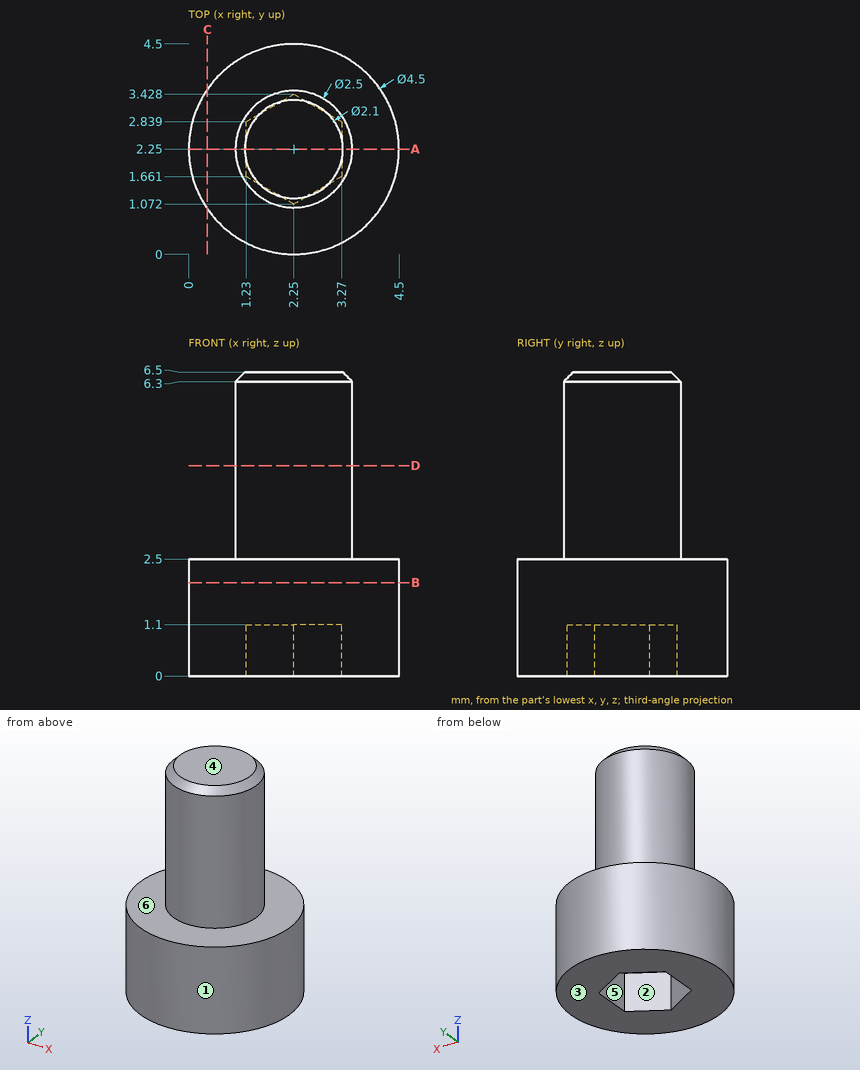
Can you work these out from the drawing? Everything is in mm from the part's minimum corner. A direction names the side the tool comes from. Round coordinates to 2 decimals unless told otherwise and drop trailing zeros. Write each loop counter-clockwise with the first axis right and the second up, starting at its lowest first coordinate (ties: lowest second). Pieces come first, ordered by that corner, then holes. Notation, with made-up numbers: (2, 63.5) - (28, 63.5) arc R24 ccw to (28, 75.5) - close; hole circle Ø10 at (-39.75, 57). An arc over 180 degrees is marked (long way). Write each question's results on one line, items separated by ' | '. Start each with the question number.
1) Suppose I cut it at B-B (z = 2). List the corners of the cut face in (x, y) for me.
2) Suppose I cut it at A-A (y = 2.25). List the corners of the cut face in (x, z) for me.
3) Suppose I cut it at D-D (z = 4.5). List the corners of the cut face in (x, y) for me, and give its area (3 significant figures).
4) Which directions (+Z, -Z, +X, -X, +Y, -Y) give clear straight access to the entire face, cutting with the end or side of a thin tool? Please do the marked faces 4, 5 and 6.
5) Please list where these lines run through material, in increasing order: line 1 (Y direction, x = 1.6, z = 1); line 2 (Z direction, x = 3.8, y = 3); line 3 (X direction, y = 1.95, z = 0.5).
6) We'd pull the mould along Y, two halves only. Please class the marked faces 1, 2 and 3: released by +Y, released by -Y, zero draft, split by the parting line, or undercut.
7) For pin 1 Ø2 at (x, z) = (0.5, 4) entering from +Y, with a flat end and sliding along its axis, tell me the tip position at first contact or that it passes through.
8) Suppose I cut it at C-C (x = 0.4). List the corners of the cut face in (y, z) for me.
Here are the results:
1) outline: circle Ø4.5 at (2.25, 2.25)
2) outline: (0, 0) - (1.23, 0) - (1.23, 1.1) - (3.27, 1.1) - (3.27, 0) - (4.5, 0) - (4.5, 2.5) - (3.5, 2.5) - (3.5, 6.3) - (3.3, 6.5) - (1.2, 6.5) - (1, 6.3) - (1, 2.5) - (0, 2.5) - close
3) outline: circle Ø2.5 at (2.25, 2.25) | area: 4.91 mm2
4) face 4: +Z, +X, -X, +Y, -Y | face 5: -Z | face 6: +Z
5) line 1: y = 0.1 to 1.45, 3.05 to 4.4 | line 2: z = 0 to 2.5 | line 3: x = 0.02 to 1.23, 3.27 to 4.48
6) face 1: split by the parting line | face 2: undercut | face 3: zero draft
7) pin 1: stops at y = 3.25
8) outline: (0.97, 0) - (3.53, 0) - (3.53, 2.5) - (0.97, 2.5) - close
